```python
from build123d import *

# Parameters (mm, degrees)
BOSS_EXTRUDE1_DEPTH = 97.62
SKETCH2_W           = 4
SKETCH2_H           = 6.25
SKETCH2_W_2         = 6.25
SKETCH2_H_2         = 4
CUT_EXTRUDE1_DEPTH  = 3
SKETCH5_W           = 25
SKETCH5_H           = 9
BOSS_EXTRUDE4_DEPTH = 3


with BuildPart() as part:
    # Sketch1 → Boss-Extrude1 (new body)
    with BuildSketch(Plane(origin=(0, 0, 0), x_dir=(1, 0, 0), z_dir=(0, 1, 0))):
        with BuildLine():
            Line((-32.735485333, 2.21), (-35.741740305, 2.21))
            ThreePointArc((-35.741740305, 2.21), (-34.793989799, -8.469614742), (-30.727251748, -18.39))
            Line((-30.727251748, -18.39), (-27.171750036, -18.39))
            ThreePointArc((-27.171750036, -18.39), (-31.675056628, -8.554933525), (-32.735485333, 2.21))
        make_face()
        with BuildLine():
            ThreePointArc((35.81, 0), (35.792931008, 1.105526954), (35.741740305, 2.21))
            Line((35.741740305, 2.21), (32.735485333, 2.21))
            ThreePointArc((32.735485333, 2.21), (32.791366042, 1.105627925), (32.81, 0))
            ThreePointArc((32.81, 0), (31.368783995, -9.617457599), (27.171750036, -18.39))
            Line((27.171750036, -18.39), (30.727251748, -18.39))
            ThreePointArc((30.727251748, -18.39), (34.515930996, -9.539738332), (35.81, 0))
        make_face()
        with BuildLine():
            ThreePointArc((-30.727251748, -18.39), (-29.761325298, -19.915311108), (-28.719749303, -21.39))
            Line((-28.719749303, -21.39), (-24.878987118, -21.39))
            ThreePointArc((-24.878987118, -21.39), (-26.06855979, -19.923009071), (-27.171750036, -18.39))
            Line((-27.171750036, -18.39), (-30.727251748, -18.39))
        make_face()
        with BuildLine():
            Line((24.878987118, -21.39), (28.719749303, -21.39))
            ThreePointArc((28.719749303, -21.39), (29.761325298, -19.915311108), (30.727251748, -18.39))
            Line((30.727251748, -18.39), (27.171750036, -18.39))
            ThreePointArc((27.171750036, -18.39), (26.06855979, -19.923009071), (24.878987118, -21.39))
        make_face()
        with BuildLine():
            ThreePointArc((-27.171750036, -18.39), (-26.06855979, -19.923009071), (-24.878987118, -21.39))
            Line((-24.878987118, -21.39), (24.878987118, -21.39))
            ThreePointArc((24.878987118, -21.39), (26.06855979, -19.923009071), (27.171750036, -18.39))
            Line((27.171750036, -18.39), (-27.171750036, -18.39))
        make_face()
        with BuildLine():
            Line((-32.393703092, 5.21), (-35.428971196, 5.21))
            ThreePointArc((-35.428971196, 5.21), (-35.616955848, 3.713294511), (-35.741740305, 2.21))
            Line((-35.741740305, 2.21), (-32.735485333, 2.21))
            ThreePointArc((-32.735485333, 2.21), (-32.59912263, 3.713933733), (-32.393703092, 5.21))
        make_face()
        with BuildLine():
            ThreePointArc((35.741740305, 2.21), (35.616955848, 3.713294511), (35.428971196, 5.21))
            Line((35.428971196, 5.21), (32.393703092, 5.21))
            ThreePointArc((32.393703092, 5.21), (32.59912263, 3.713933733), (32.735485333, 2.21))
            Line((32.735485333, 2.21), (35.741740305, 2.21))
        make_face()
        with BuildLine():
            Line((32.393703092, 5.21), (-32.393703092, 5.21))
            ThreePointArc((-32.393703092, 5.21), (-32.59912263, 3.713933733), (-32.735485333, 2.21))
            Line((-32.735485333, 2.21), (32.735485333, 2.21))
            ThreePointArc((32.735485333, 2.21), (32.59912263, 3.713933733), (32.393703092, 5.21))
        make_face()
        with BuildLine():
            Line((-32.393703092, 5.21), (-35.428971196, 5.21))
            ThreePointArc((-35.428971196, 5.21), (-35.616955848, 3.713294511), (-35.741740305, 2.21))
            Line((-35.741740305, 2.21), (-32.735485333, 2.21))
            ThreePointArc((-32.735485333, 2.21), (-32.59912263, 3.713933733), (-32.393703092, 5.21))
        make_face()
        with BuildLine():
            ThreePointArc((35.741740305, 2.21), (35.616955848, 3.713294511), (35.428971196, 5.21))
            Line((35.428971196, 5.21), (32.393703092, 5.21))
            ThreePointArc((32.393703092, 5.21), (32.59912263, 3.713933733), (32.735485333, 2.21))
            Line((32.735485333, 2.21), (35.741740305, 2.21))
        make_face()
        with BuildLine():
            Line((-32.735485333, 2.21), (-35.741740305, 2.21))
            ThreePointArc((-35.741740305, 2.21), (-34.793989799, -8.469614742), (-30.727251748, -18.39))
            Line((-30.727251748, -18.39), (-27.171750036, -18.39))
            ThreePointArc((-27.171750036, -18.39), (-31.675056628, -8.554933525), (-32.735485333, 2.21))
        make_face()
        with BuildLine():
            ThreePointArc((35.81, 0), (35.792931008, 1.105526954), (35.741740305, 2.21))
            Line((35.741740305, 2.21), (32.735485333, 2.21))
            ThreePointArc((32.735485333, 2.21), (32.791366042, 1.105627925), (32.81, 0))
            ThreePointArc((32.81, 0), (31.368783995, -9.617457599), (27.171750036, -18.39))
            Line((27.171750036, -18.39), (30.727251748, -18.39))
            ThreePointArc((30.727251748, -18.39), (34.515930996, -9.539738332), (35.81, 0))
        make_face()
        with BuildLine():
            ThreePointArc((-30.727251748, -18.39), (-29.761325298, -19.915311108), (-28.719749303, -21.39))
            Line((-28.719749303, -21.39), (-24.878987118, -21.39))
            ThreePointArc((-24.878987118, -21.39), (-26.06855979, -19.923009071), (-27.171750036, -18.39))
            Line((-27.171750036, -18.39), (-30.727251748, -18.39))
        make_face()
        with BuildLine():
            Line((24.878987118, -21.39), (28.719749303, -21.39))
            ThreePointArc((28.719749303, -21.39), (29.761325298, -19.915311108), (30.727251748, -18.39))
            Line((30.727251748, -18.39), (27.171750036, -18.39))
            ThreePointArc((27.171750036, -18.39), (26.06855979, -19.923009071), (24.878987118, -21.39))
        make_face()
    extrude(amount=BOSS_EXTRUDE1_DEPTH)

    # Sketch2 → Cut-Extrude1 (cut)
    with BuildSketch(Plane(origin=(-23.61, 0, 21.39), x_dir=(-1, 0, 0), z_dir=(0, 0, -1))):
        with Locations((1.550812332, 63.125)):
            Rectangle(SKETCH2_W, SKETCH2_H)
        with Locations((-14.449187668, 33.125)):
            Rectangle(SKETCH2_W, SKETCH2_H)
        with Locations((-14.449187668, 63.125)):
            Rectangle(SKETCH2_W, SKETCH2_H)
        with Locations((-19.832327081, 89)):
            Rectangle(SKETCH2_W_2, SKETCH2_H_2)
        with Locations((-45.066048255, 89)):
            Rectangle(SKETCH2_W_2, SKETCH2_H_2)
        with Locations((-48.449187668, 63.125)):
            Rectangle(SKETCH2_W, SKETCH2_H)
        with Locations((-45.066048255, 11)):
            Rectangle(SKETCH2_W_2, SKETCH2_H_2)
        with Locations((-19.832327081, 11)):
            Rectangle(SKETCH2_W_2, SKETCH2_H_2)
        with Locations((1.550812332, 33.125)):
            Rectangle(SKETCH2_W, SKETCH2_H)
        with Locations((-48.449187668, 33.125)):
            Rectangle(SKETCH2_W, SKETCH2_H)
    extrude(amount=CUT_EXTRUDE1_DEPTH, mode=Mode.SUBTRACT)

    # Sketch5 → Boss-Extrude4 (add)
    with BuildSketch(Plane(origin=(0, 97.62, 0), x_dir=(1, 0, 0), z_dir=(0, 1, 0))):
        with BuildLine():
            Line((35.428971196, 5.21), (-35.428971196, 5.21))
            ThreePointArc((-35.428971196, 5.21), (-34.722537139, -8.757940089), (-28.719749303, -21.39))
            Line((-28.719749303, -21.39), (28.719749303, -21.39))
            ThreePointArc((28.719749303, -21.39), (34.722537139, -8.757940089), (35.428971196, 5.21))
        make_face()
        with Locations((-14.660228428, -13.89)):
            Rectangle(SKETCH5_W, SKETCH5_H, mode=Mode.SUBTRACT)
        with Locations((14.660228428, -13.89)):
            Rectangle(SKETCH5_W, SKETCH5_H, mode=Mode.SUBTRACT)
    extrude(amount=BOSS_EXTRUDE4_DEPTH)


solid = part.part
```
Check sheet for the modelled part. Datum: model origin and axes. Units: mm. A direction names the side the tool comes from. Coordinates: 2 decimals unless noted, no trailing zeros. Order: outer loops, then holes, each group sorted by start corner. A loop starts at its lowest first (then second) coordinate and runs counter-clockwise, first axis right, second up. Notation, with made-up numbers: M 6,33 L 33,33 A24 ccw 33,60 Z; hole C 86.25,21.25 d2. An arc over 180 degrees is marked long. One line per question, with ' | ' between items. Start each with the question number.
Item 1: Mould release check, pull along Z, two halves, no side actions. Record for faces 1 (the flat face through (0, 50, 18.39)), 2 (the cylindrical face through (-31.635, 48.127, 8.702)), 3 (the flat face through (-27.161, 63, 20)): pulls with the +Z half, pulls with the -Z half, needs draft (parallel to the pull), parting line crosses it, or undercut.
Item 2: Sectioned sample at C-C on z = 11.25. Record the cut outline in (x, y).
Item 3: Material ranges on line 1 (Z direction, x = 11.5, y = 90); line 2 (X direction, y = 72, z = 1); line 3 (Y direction, x = 8, z = 5.75), recorded low to high.
Item 4: Sectioned sample at D-D on x = 17. Record the cut outline in (y, z).
Item 5: Sectioned sample at B-B on y = 63. Count the separate pieces of the cut face and the enclosed holes in it, and give its area (3 significant figures).
Item 6: Access from +Z, -Z, +X, -X, +Y, -Y to the whole of each face (thin tool, end or side, straight path). Record for faces 4 (the flat face through (24.581, 89, 20)), 5 (the flat face through (0, 0, -3)), 6 (the flat face through (0, 48, -2.21)).
Item 7: Gauge pin test, flat ends, axial feed: P1, Ø1.5, axis at y = 64.5, z = 20.5, coming from the +X side; P2, Ø2.5, axis at y = 62, z = 20.5, coming from the -X side; P3, Ø0.9, axis at y = 11.5, z = 20, coming from the -X side. Record the tip position at first contact, or that the pin passes through.
Item 8: Sectioned sample at A-A on x = -25. Record the cut outline in (y, z), and give its area (3 significant figures).
Answer below:
1) face 1: undercut | face 2: undercut | face 3: needs draft
2) outline: M -34,0 L -30.82,0 L -30.82,97.62 L -27.16,97.62 L -27.16,100.62 L -34,100.62 Z; M -2.16,97.62 L 2.16,97.62 L 2.16,100.62 L -2.16,100.62 Z; M 27.16,97.62 L 30.82,97.62 L 30.82,0 L 34,0 L 34,100.62 L 27.16,100.62 Z
3) line 1: z = -5.21 to -2.21, 18.39 to 21.39 | line 2: x = -35.8 to -32.79, 32.79 to 35.8 | line 3: y = 97.62 to 100.62
4) outline: M 0,-5.21 L 100.62,-5.21 L 100.62,9.39 L 97.62,9.39 L 97.62,-2.21 L 0,-2.21 Z; M 0,18.39 L 100.62,18.39 L 100.62,21.39 L 0,21.39 Z
5) separate pieces: 3 | enclosed holes: 0 | area: 486 mm^2
6) face 4: +Z | face 5: +Z, -Z, +X, -X, -Y | face 6: -Y
7) P1: stops at x = 29.87 | P2: stops at x = -30.2 | P3: stops at x = -30
8) outline: M 0,-5.21 L 100.62,-5.21 L 100.62,9.39 L 97.62,9.39 L 97.62,-2.21 L 0,-2.21 Z; M 0,18.39 L 30,18.39 L 30,21.39 L 0,21.39 Z; M 36.25,18.39 L 60,18.39 L 60,21.39 L 36.25,21.39 Z; M 66.25,18.39 L 100.62,18.39 L 100.62,21.39 L 66.25,21.39 Z | area: 601 mm^2
